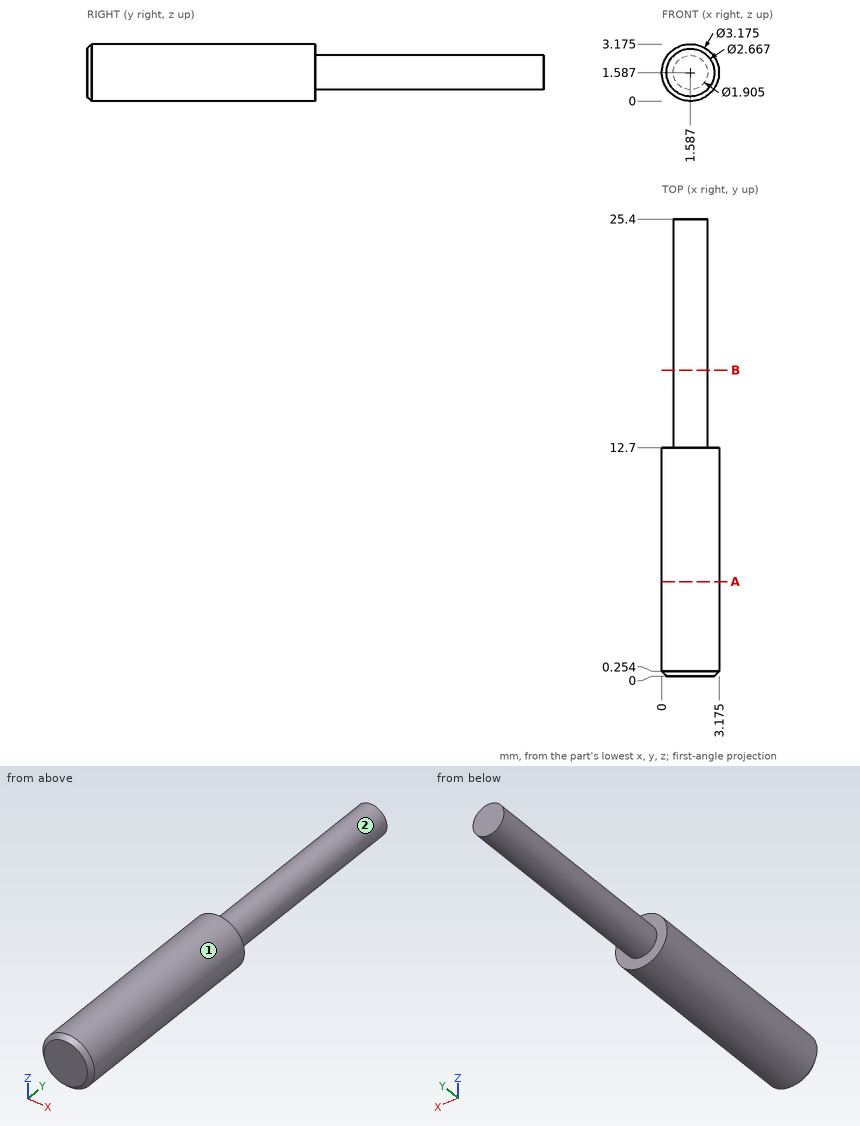
Answer from the drawing. Dimensions are ordinates in mm from the lowest x, y and z of the part. A direction names the side the tool comes from. Round coordinates to 2 decimals unless told otherwise and drop trailing zeros. Loops run counter-clockwise (first coordinate to the right, second up) from the corner with the lowest first, then second, coordinate; pieces in that order, holes last.
(1) Find the intervals of material crossed by L1, parallel to Z at x = 1.5, y = 4.75; L2, parallel to Y at x = 2.6, z = 1; L3, parallel to Z at x = 0.6, y = 8.5 (1 decimal), in increasing order.
Computed values:
L1: z = 0 to 3.17
L2: y = 0 to 12.7
L3: z = 0.3 to 2.8
(2) For the marked faces 1 and 2, determine the directions among +Z, -Z, +X, -X, +Y, -Y from which every point of the face is accessible in a straight line to the end or side of a thin tool.
Computed values:
face 1: +Y, -Y
face 2: +Y
(3) The part is cut by section B-B, the plane y = 17. Give the vertices of the cut face in (x, z) (1 decimal).
Computed values:
outline: circle Ø1.9 at (1.6, 1.6)
(4) The part is cut by section A-A, the plane y = 5.25. Give the vertices of the cut face in (x, z) (1 decimal).
Computed values:
outline: circle Ø3.2 at (1.6, 1.6)
